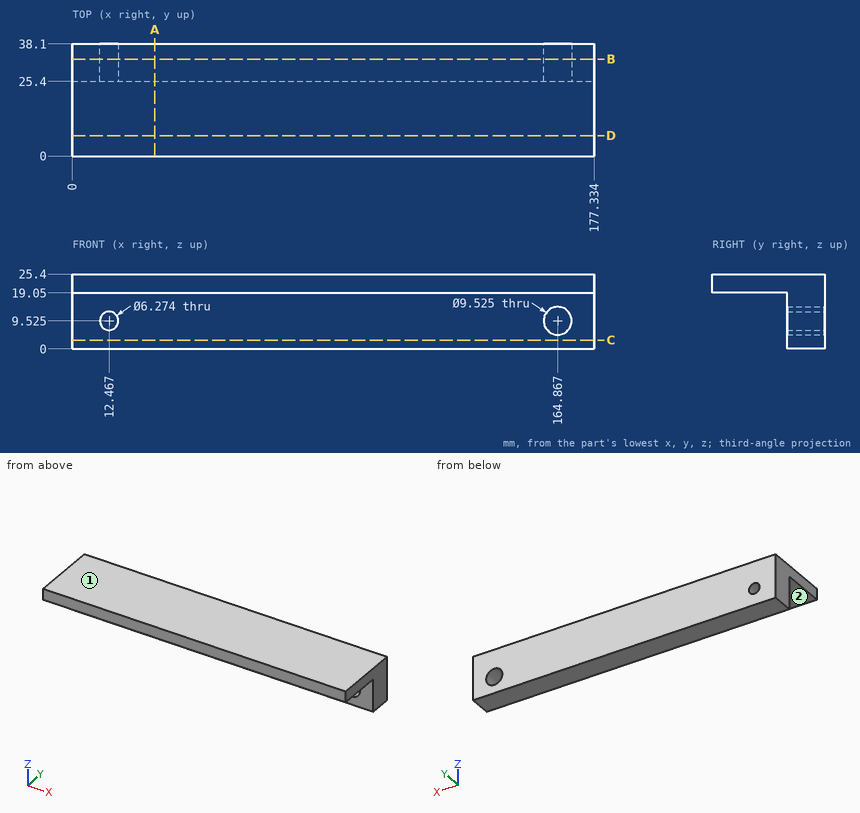
Geometry check sheet. Reference: drawing and pictorial views, mm from the part's lowest x, y, z. A direction names the side the tool comes from. Give positions to 0.01 mm unless a question says otherwise; leave off trailing zeros. Order: outer loops, then holes, each group sorted by start corner. A loop starts at its lowest first (then second) coordinate and runs counter-clockwise, first axis right, second up. Notation, with made-up numbers: (48.5, 72) - (64.5, 72) arc R24 ccw to (64.5, 110) - close; hole circle Ø7 at (-9.5, 21.5). An arc over 180 degrees is marked (long way). Use one line per item in the form item = value.
1) Sectioned sample at A-A (x = 28). Record the boundary of the cut face in (y, z), and give its area (3 significant figures).
Working result:
outline = (0, 19.05) - (25.4, 19.05) - (25.4, 0) - (38.1, 0) - (38.1, 25.4) - (0, 25.4) - close
area = 484 mm^2
2) Material ranges on probe 1 along X at (y, z) = (34, 11) (1 decimal); probe 2 along Z at (x, y) = (75, 3.5); probe 3 along Y at (x, z) = (153, 1.5), recorded low to high. Write a range as from..to.
Working result:
probe_1 = 0..9.7, 15.2..160.3, 169.4..177.3
probe_2 = 19.05..25.4
probe_3 = 25.4..38.1
3) Sectioned sample at B-B (y = 33). Record the boundary of the cut face in (x, z) (1 decimal).
Working result:
outline = (0, 0) - (177.3, 0) - (177.3, 25.4) - (0, 25.4) - close; hole circle Ø6.3 at (12.5, 9.5); hole circle Ø9.5 at (164.9, 9.5)
4) Sectioned sample at C-C (z = 3). Record the boundary of the cut face in (x, y), and give its area (3 significant figures).
Working result:
outline = (0, 25.4) - (177.33, 25.4) - (177.33, 38.1) - (0, 38.1) - close
area = 2,250 mm^2
5) Sectioned sample at D-D (y = 7). Record the boundary of the cut face in (x, z), and give its area (3 significant figures).
Working result:
outline = (0, 19.05) - (177.33, 19.05) - (177.33, 25.4) - (0, 25.4) - close
area = 1,130 mm^2
6) Access from +Z, -Z, +X, -X, +Y, -Y to the whole of each face (thin tool, end or side, straight path). Record for the marked faces 1 and 2.
Working result:
face_1 = +Z, +X, -X, +Y, -Y
face_2 = -Z, +X, -X, -Y
7) Depth check by flat-ended pin: pin 1 Ø10 at (x, z) = (12.467, 9.525) entering from +Y; pin 2 Ø1.5 at (x, y) = (32.5, 18) entering from -Z; pin 3 Ø1 at (x, z) = (151, 16.5) entering from -Y; pin 4 Ø7.5 at (x, z) = (164.867, 9.525) entering from -Y. Enter the tip coordinate at first touch or a pass-through.
Working result:
pin_1 = 38.1
pin_2 = 19.05
pin_3 = 25.4
pin_4 = through
